Autodesk Fusion 360 part; units mm, degrees
sketch "Sketch1" plane through (0, 0, 0) normal (0, 0, 1) x (1, 0, 0)
  line L0 (0, 0) -> (37, 0)
  line L1 (37, 0) -> (37, 25)
  line L2 (37, 25) -> (0, 25)
  line L3 (0, 25) -> (0, 0)
  dimension "d1" = 37
  dimension "d2" = 25
extrude "Extrude1" add sketch "Sketch1" along normal blind 2
sketch "Sketch2" plane through (0, 0, 2) normal (0, 0, 1) x (-1, 0, 0)
  line L0 (0, -25) -> (0, 0)
  line L1 (0, 0) -> (-37, 0)
  line L2 (-37, 0) -> (-37, -25)
  line L3 (-37, -25) -> (0, -25)
  line L4 (0, -25) -> (-2, -25)
  line L5 (-2, -25) -> (-2, 0)
  line L6 (-2, 0) -> (0, 0)
  line L7 (0, 0) -> (0, -25)
  line L8 (-37, -25) -> (-35, -25)
  line L9 (-35, -25) -> (-35, 0)
  line L10 (-35, 0) -> (-37, 0)
  line L11 (-37, 0) -> (-37, -25)
  dimension "d5" = 2
  dimension "d6" = 25
  dimension "d7" = 2
  dimension "d8" = 25
extrude "Extrude2" add sketch "Sketch2" along normal blind 16 contours L0 L1 L3 L4 L5 L6 L7 | L1 L2 L3 L8 L9 L10 L11
sketch "Sketch3" plane through (0, 0, 18) normal (0, 0, 1) x (-1, 0, 0)
  line L0 (-37, 0) -> (-37, -25)
  line L1 (-37, -25) -> (-35, -25)
  line L2 (-35, -25) -> (-35, 0)
  line L3 (-35, 0) -> (-37, 0)
  line L4 (0, -25) -> (-37, -25)
  line L5 (-37, -25) -> (-37, 0)
  line L6 (-37, 0) -> (0, 0)
  line L7 (0, 0) -> (0, -25)
extrude "Extrude3" add sketch "Sketch3" along normal blind 20
sketch "Sketch4" plane through (0, 0, 0) normal (0, -1, 0) x (1, 0, 0)
  line L0 (0, 38) -> (0, 0)
  line L1 (0, 0) -> (37, 0)
  line L2 (37, 0) -> (37, 38)
  line L3 (37, 38) -> (0, 38)
  line L4 (2, 18) -> (35, 18)
  line L5 (35, 18) -> (35, 2)
  line L6 (35, 2) -> (2, 2)
  line L7 (2, 2) -> (2, 18)
  line L8 (0, 20) -> (37, 22)
extrude "Extrude4" cut sketch "Sketch4" against normal blind 40 contours L0 L2 L3 L8
sketch "Sketch5" plane through (-1.0779, 0, 19.9417) normal (-0.054, 0, 0.9985) x (0, -1, 0)
  line L0 (-25, 38.1335) -> (-25, 1.0795)
  line L1 (-25, 1.0795) -> (0, 1.0795)
  line L2 (0, 1.0795) -> (0, 38.1335)
  line L3 (0, 38.1335) -> (-25, 38.1335)
  line L4 (-25, 1.0795) -> (-12.5, 1.0795)
  line L5 (-12.5, 1.0795) -> (-12.5, 19.5795)
  line L6 (-12.5, 19.5795) -> (-25, 19.5795)
  line L7 (-25, 19.5795) -> (-25, 1.0795)
  circle A0 centre (-12.5, 19.5795) radius 10
  dimension "d15" = 12.5
  dimension "d16" = 18.5
  dimension "d17" = 20
extrude "Extrude5" cut sketch "Sketch5" against normal blind 2 contours L5 L6 A0 | L5 L6 A0
extrude "Extrude6" add 1 faces at (24, 8.3333, 18) along direction (0, 0, -1) blind 1
Can you work these out from the model? Positions are in its coordinate system, mm. A direction names the side the tool comes from. Give positions to 0.01 mm unless a question says otherwise; leave off trailing zeros. Loops run counter-clockwise (first coordinate to the right, second up) from the corner with the lowest first, then second, coordinate; pieces in that order, holes last. Notation, with made-up numbers: (-27.5, 40) -> (28.5, 40) arc R15 cw to (28.5, 53) -> close; hole circle Ø1 at (-23.5, -25). An arc over 180 degrees is marked (long way). Return JSON: item names as keys, results as strings.
Q1. I need wall thicknesses on probe 1 along X at (y, z) = (7, 12); probe 2 along Z at (x, y) = (5, 1); probe 3 along Z at (x, y) = (9.5, 14.25). Which ranges of each line are inside material? Lowest first, please.
Checks:
{"probe 1": "x = 0 to 2, 35 to 37", "probe 2": "z = 0 to 2, 17 to 20.27", "probe 3": "z = 0 to 2, 17 to 18.51"}
Q2. We'd pull the mould along Z, two halves only. Please class faces 1 (the face through (18, 13, 2)), 2 (the face through (0, 13, 10)), 3 (the face through (18, 13, 0)): released by +Z, released by -Z, zero draft, split by the parting line, or undercut.
Checks:
{"face 1": "undercut", "face 2": "zero draft", "face 3": "released by -Z"}
Q3. I want a section at B-B, the plane y = 20.75. List the corners of the cut face in (x, z) for me.
Checks:
{"outline": "(0, 0) -> (37, 0) -> (37, 22) -> (24.12, 21.3) -> (24.22, 19.31) -> (12.94, 18.7) -> (12.83, 20.69) -> (0, 20) -> close; hole (2, 2) -> (35, 2) -> (35, 17) -> (2, 17) -> close"}
Q4. I want a section at C-C, the plane x = 6. List the corners of the cut face in (y, z) for me.
Checks:
{"outline": "(0, 0) -> (25, 0) -> (25, 2) -> (0, 2) -> close; (0, 17) -> (25, 17) -> (25, 20.32) -> (0, 20.32) -> close"}
Q5. I want a section at D-D, the plane y = 16.25. List the corners of the cut face in (x, z) for me, then the cut area to 3 significant figures.
Checks:
{"outline": "(0, 0) -> (37, 0) -> (37, 22) -> (27.73, 21.5) -> (27.84, 19.5) -> (9.32, 18.5) -> (9.22, 20.5) -> (0, 20) -> close; hole (2, 2) -> (35, 2) -> (35, 17) -> (2, 17) -> close", "area": "245 mm2"}
Q6. I want a section at A-A, the plane z = 7. List the corners of the cut face in (x, y) for me, then the cut area to 3 significant figures.
Checks:
{"outline": "(0, 0) -> (2, 0) -> (2, 25) -> (0, 25) -> close; (35, 0) -> (37, 0) -> (37, 25) -> (35, 25) -> close", "area": "100 mm2"}
Q7. For pin 1 Ø4 at (x, y) = (22.5, 16) entering from +Z; pin 2 Ø1 at (x, y) = (30.5, 13) entering from +Z; pin 3 Ø7.5 at (x, y) = (26, 15.5) entering from +Z, each with a flat end and sliding along its axis, tell me the tip position at first contact or that it passes through.
Checks:
{"pin 1": "stops at z = 19.32", "pin 2": "stops at z = 21.68", "pin 3": "stops at z = 21.61"}
Q8. On a 3-axis mill with a long thin cutter (end or side, diameter ignored), from which of +Z, -Z, +X, -X, +Y, -Y can I reach the whole of each face in a straight line? I mean faces 4 (the face through (18, 0, 18)), 5 (the face through (19, 12, 17)). Say none if no direction works.
Checks:
{"face 4": "+Z, -Z, +X, -X, -Y", "face 5": "+Y, -Y"}
